CAD build for the part. Positions are in the model's coordinates, mm. Coordinates: 2 decimals unless noted, no trailing zeros. Write each loop counter-clockwise with the first axis right and the second up, starting at its lowest first coordinate (ties: lowest second). Pieces come first, ordered by that corner, then holes. Notation, with made-up numbers: (48, 0) -> (105, 0) arc R18 ccw to (105, 23) -> close; hole circle Ø7 at (15.5, 53). An arc over 180 degrees is marked (long way). Answer as CSV lines item,"result". Start each with the question number.
```python
from build123d import *

# Parameters (mm, degrees)
SKETCH4_W           = 25.4
SKETCH4_H           = 25.4
SKETCH4_W_2         = 23
SKETCH4_H_2         = 23
SKETCH5_W           = 25.4
SKETCH5_H           = 25.4
SKETCH5_W_2         = 23
SKETCH5_H_2         = 23
BOSS_EXTRUDE2_DEPTH = 253.8


with BuildPart() as part:
    # Sweep1: sweep along a path in Sketch3
    with BuildLine(Plane.XY) as sweep1_path:
        Line((-250, -304.6), (250, -304.6))
        Line((250, -304.6), (450, -104.6))
        Line((450, -104.6), (450, 0))
        Line((450, 0), (-450, 0))
        Line((-450, 0), (-450, -104.6))
        Line((-450, -104.6), (-250, -304.6))
    # Sketch4 → Sweep1 (sweep)
    with BuildSketch(Plane(origin=(0, 0, 0), x_dir=(0, 0, -1), z_dir=(1, 0, 0))):
        with Locations((12.7, -291.9)):
            Rectangle(SKETCH4_W, SKETCH4_H)
        with Locations((12.7, -291.9)):
            Rectangle(SKETCH4_W_2, SKETCH4_H_2, mode=Mode.SUBTRACT)
    sweep(path=sweep1_path.line, transition=Transition.RIGHT)

    # Sketch5 → Boss-Extrude2 (add)
    with BuildSketch(Plane(origin=(-272.712994231, -279.2, 0), x_dir=(-1, 0, 0), z_dir=(0, 1, 0))):
        with Locations((-360.012994231, -12.7)):
            Rectangle(SKETCH5_W, SKETCH5_H)
        with Locations((-360.012994231, -12.7)):
            Rectangle(SKETCH5_W_2, SKETCH5_H_2, mode=Mode.SUBTRACT)
        with Locations((-185.412994231, -12.7)):
            Rectangle(SKETCH5_W, SKETCH5_H)
        with Locations((-185.412994231, -12.7)):
            Rectangle(SKETCH5_W_2, SKETCH5_H_2, mode=Mode.SUBTRACT)
    extrude(amount=BOSS_EXTRUDE2_DEPTH)


solid = part.part
```
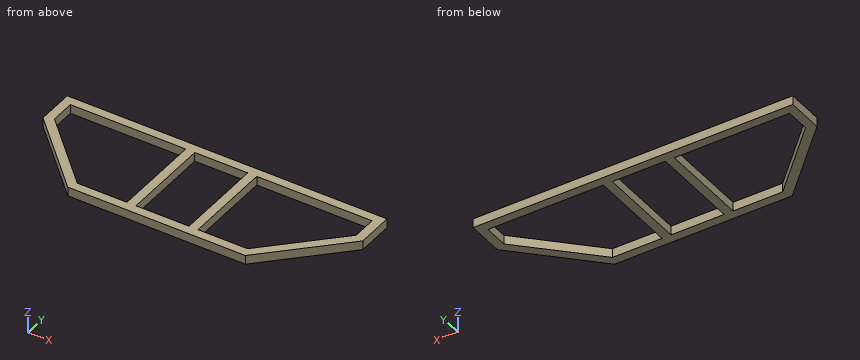
1. Cut at A-A (x = 163.5). Give the cut face in (y, z), then the cut area to 3 significant figures.
2. Flat gauge pins, fed straight in: P1, Ø3, axis at y = -181, z = -10, coming from the -X side; P2, Ø2, axis at y = -113, z = -13.5, coming from the +X side; P3, Ø12.5, axis at x = -260, z = -16.5, coming from the -Y side; P4, Ø12.5, axis at y = -106.5, z = -7, coming from the -X side. Where does each tip first touch, or does it go through?
3. Wall check: line 1 (Y direction, x = -184, z = -21); line 2 (Y direction, x = -356, z = -19.25); line 3 (X direction, y = -14.5, z = -5.25). Give the ranges that are in metal, low to high.
4. Cut at B-B (y = -49.5). Count the separate pieces of the cut face and the enclosed holes in it, then the cut area to 3 significant figures.
5. Cut at D-D (x = 396). Give the cut face in (y, z).
Geometry check:
1,outline,"(-304.6, -25.4) -> (-279.2, -25.4) -> (-279.2, 0) -> (-304.6, 0) -> close; (-25.4, -25.4) -> (0, -25.4) -> (0, 0) -> (-25.4, 0) -> close; hole (-303.4, -24.2) -> (-280.4, -24.2) -> (-280.4, -1.2) -> (-303.4, -1.2) -> close; hole (-24.2, -24.2) -> (-1.2, -24.2) -> (-1.2, -1.2) -> (-24.2, -1.2) -> close"
1,area,"232 mm²"
2,P1,"x = -375.1"
2,P2,"x = 442.6"
2,P3,"y = -300.85"
2,P4,"x = -450"
3,line 1,"-304.6 to -303.4, -280.4 to -279.2, -25.4 to -24.2, -1.2 to 0"
3,line 2,"-198.6 to -196.9, -164.38 to -162.68, -25.4 to -24.2, -1.2 to 0"
3,line 3,"-450 to -448.8, 448.8 to 450"
4,separate pieces,"4"
4,enclosed holes,"4"
4,area,"465 mm²"
5,outline,"(-158.6, -25.4) -> (-122.68, -25.4) -> (-122.68, 0) -> (-158.6, 0) -> close; (-25.4, -25.4) -> (0, -25.4) -> (0, 0) -> (-25.4, 0) -> close; hole (-156.9, -24.2) -> (-124.38, -24.2) -> (-124.38, -1.2) -> (-156.9, -1.2) -> close; hole (-24.2, -24.2) -> (-1.2, -24.2) -> (-1.2, -1.2) -> (-24.2, -1.2) -> close"
